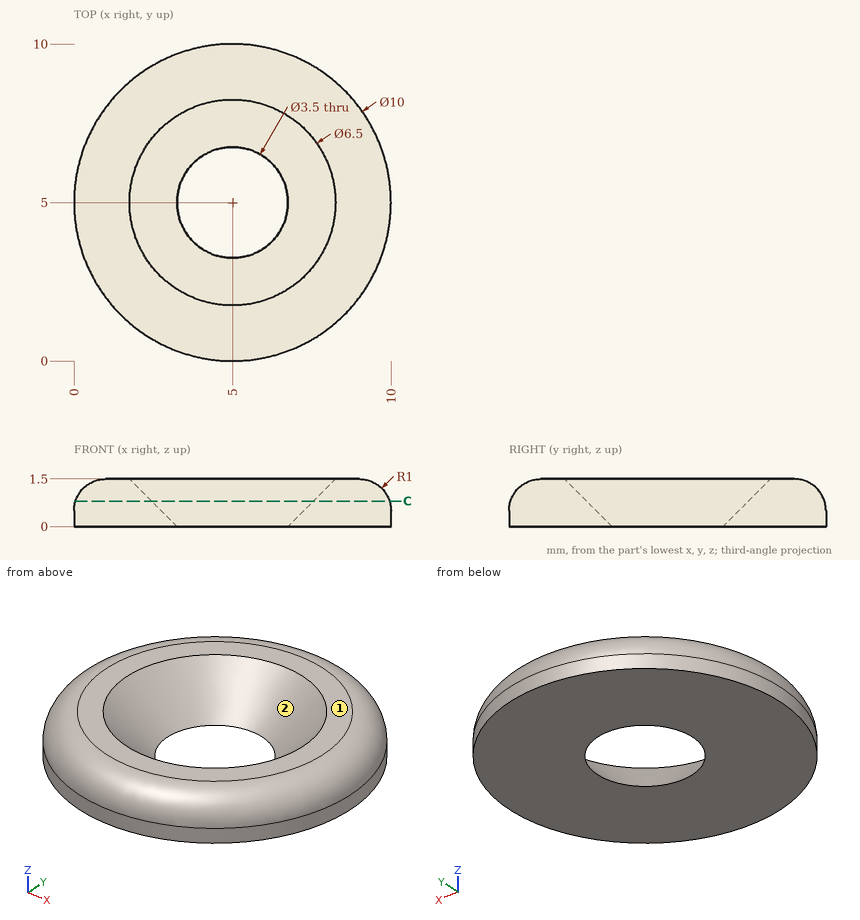
For this review, use the dimensioned drawing (mm, ordinates from the lowest corner) and the shaded views. Coordinates: 2 decimals unless noted, no trailing zeros. Loops run counter-clockwise (first coordinate to the right, second up) from the corner with the lowest first, then second, coordinate; pieces in that order, holes last.
1. Insertion check: P1, Ø2, axis at x = 5, y = 5, coming from the +Z side. The pin has a flat end and moves straight along its axis. Give the tip position at first contact, or say it passes through.
2. For line 1 (X direction, y = 3.25, z = 0.9) (1 decimal); line 2 (X direction, y = 6, z = 1.05) (1 decimal); line 3 (Y direction, x = 4.5, z = 0.8), list the stretches that pass through material, from the lowest coordinate up.
3. Add section C-C, the plane z = 0.8. Give the boundary of the cut face in (x, y).
4. Mouldability with a two-part tool opening along Y and no side actions: class the marked faces 1 and 2 as +Y half, -Y half, draft (parallel to the pull), parting line (faces both ways), or undercut.
Result:
1. P1: passes through
2. line 1: x = 0.4 to 3, 7 to 9.6
2. line 2: x = 0.3 to 2.4, 7.6 to 9.7
2. line 3: y = 0.07 to 2.5, 7.5 to 9.93
3. outline: circle Ø9.91 at (5, 5); hole circle Ø5.1 at (5, 5)
4. face 1: draft
4. face 2: undercut
